The listing builds one solid part. Answer for the finished solid, in the listing's coordinates (mm). A direction names the side the tool comes from. Round coordinates to 2 decimals unless told otherwise and drop trailing zeros. Order: outer loops, then holes, each group sorted by start corner. A loop starts at its lowest first (then second) coordinate and runs counter-clockwise, first axis right, second up. Notation, with made-up numbers: (40, 31) -> (91, 31) arc R15 cw to (91, 46) -> close; hole circle Ø11 at (40, -1.75). An arc over 180 degrees is marked (long way). Answer in a Markdown table with one row per item. Add a question column.
```python
from build123d import *

# Parameters (mm, degrees)
SKETCH2_R           = 1.25
BOSS_EXTRUDE1_DEPTH = 69
SKETCH3_W           = 62
SKETCH3_H           = 4.5
CUT_EXTRUDE1_DEPTH  = 113.504444357
SKETCH4_W           = 54.406446317
SKETCH4_H           = 2.417375431
BOSS_EXTRUDE2_DEPTH = 83
FILLET1_R           = 1.5
FILLET2_R           = 2.5
FILLET3_R           = 1.5
CUT_EXTRUDE3_DEPTH  = 113.504444497
CUT_EXTRUDE5_REACH  = 114.504
SKETCH7_W           = 35
SKETCH7_H           = 3.5


with BuildPart() as part:
    # Sketch2 → Boss-Extrude1 (new body)
    with BuildSketch(Plane.XY):
        Polygon((0, 0), (0, 8), (88.5, 8), (88.5, 2.5), (85, 0), align=None)
        with Locations((6.000001876, 4)):
            Circle(SKETCH2_R, mode=Mode.SUBTRACT)
        with Locations((79.120881892, 4)):
            Circle(SKETCH2_R, mode=Mode.SUBTRACT)
    extrude(amount=BOSS_EXTRUDE1_DEPTH)

    # Sketch3 → Cut-Extrude1 (cut, through all)
    with BuildSketch(Plane.ZY):
        with Locations((34.5, 5.75)):
            Rectangle(SKETCH3_W, SKETCH3_H)
    extrude(amount=-CUT_EXTRUDE1_DEPTH, mode=Mode.SUBTRACT)

    # Sketch4 → Boss-Extrude2 (add)
    with BuildSketch(Plane.ZY):
        with Locations((34.04742318, 2.291312285)):
            Rectangle(SKETCH4_W, SKETCH4_H)
    extrude(amount=-BOSS_EXTRUDE2_DEPTH)

    # Fillet1
    fillet1_edges = [part.edges().sort_by_distance(p)[0] for p in [
        (42.5, 0, 69),
        (42.5, 0, 0),
    ]]
    fillet(fillet1_edges, radius=FILLET1_R)

    # Fillet2
    # the kernel refuses this fillet: 2.5 mm, written as the material it adds along each edge
    with BuildSketch(Plane(origin=(0, 3.5, 65.5), x_dir=(0, 0, -1), z_dir=(1, 0, 0))) as fillet2_piece_1_section:
        with BuildLine():
            CenterArc((FILLET2_R, FILLET2_R), FILLET2_R, 180, 90)
            Line((0, FILLET2_R), (0, 0))
            Line((0, 0), (FILLET2_R, 0))
        make_face()
    fillet2_piece_1 = extrude(amount=11.104357952, mode=Mode.PRIVATE)
    fillet2_piece_1 = fillet2_piece_1 - Plane(origin=(6.000001876, 4, 63.653309705), x_dir=(1, 0, 0), z_dir=(0, 0, -1)) * Cylinder(1.25, 33, mode=Mode.PRIVATE)
    add(fillet2_piece_1)
    with BuildSketch(Plane(origin=(0.8956458, 3.5, 65.5), x_dir=(0, 0, -1), z_dir=(1, 0, 0))) as fillet2_piece_2_section:
        with BuildLine():
            CenterArc((FILLET2_R, FILLET2_R), FILLET2_R, 180, 90)
            Line((0, FILLET2_R), (0, 0))
            Line((0, 0), (FILLET2_R, 0))
        make_face()
    fillet2_piece_2 = extrude(amount=83.329592169, mode=Mode.PRIVATE)
    fillet2_piece_2 = fillet2_piece_2 - Plane(origin=(6.000001876, 4, 64.936218349), x_dir=(1, 0, 0), z_dir=(0, 0, -1)) * Cylinder(1.25, 177, mode=Mode.PRIVATE)
    fillet2_piece_2 = fillet2_piece_2 - Plane(origin=(79.120881892, 4, 64.936218349), x_dir=(1, 0, 0), z_dir=(0, 0, -1)) * Cylinder(1.25, 177, mode=Mode.PRIVATE)
    add(fillet2_piece_2)
    with BuildSketch(Plane(origin=(0, 3.5, 3.5), x_dir=(0, 1, 0), z_dir=(1, 0, 0))) as fillet2_piece_3_section:
        with BuildLine():
            CenterArc((FILLET2_R, FILLET2_R), FILLET2_R, 180, 90)
            Line((0, FILLET2_R), (0, 0))
            Line((0, 0), (FILLET2_R, 0))
        make_face()
    fillet2_piece_3 = extrude(amount=11.104357952, mode=Mode.PRIVATE)
    fillet2_piece_3 = fillet2_piece_3 - Plane(origin=(6.000001876, 4, 3.561814983), x_dir=(1, 0, 0), z_dir=(0, 0, -1)) * Cylinder(1.25, 33, mode=Mode.PRIVATE)
    add(fillet2_piece_3)
    with BuildSketch(Plane(origin=(74.016525816, 3.5, 3.5), x_dir=(0, 1, 0), z_dir=(1, 0, 0))) as fillet2_piece_4_section:
        with BuildLine():
            CenterArc((FILLET2_R, FILLET2_R), FILLET2_R, 180, 90)
            Line((0, FILLET2_R), (0, 0))
            Line((0, 0), (FILLET2_R, 0))
        make_face()
    fillet2_piece_4 = extrude(amount=14.483474184, mode=Mode.PRIVATE)
    fillet2_piece_4 = fillet2_piece_4 - Plane(origin=(79.120881892, 4, 4.058892955), x_dir=(1, 0, 0), z_dir=(0, 0, -1)) * Cylinder(1.25, 39, mode=Mode.PRIVATE)
    add(fillet2_piece_4)
    with BuildSketch(Plane(origin=(0.8956458, 3.5, 3.5), x_dir=(0, 1, 0), z_dir=(1, 0, 0))) as fillet2_piece_5_section:
        with BuildLine():
            CenterArc((FILLET2_R, FILLET2_R), FILLET2_R, 180, 90)
            Line((0, FILLET2_R), (0, 0))
            Line((0, 0), (FILLET2_R, 0))
        make_face()
    fillet2_piece_5 = extrude(amount=83.329592169, mode=Mode.PRIVATE)
    fillet2_piece_5 = fillet2_piece_5 - Plane(origin=(79.120881892, 4, 4.063781674), x_dir=(1, 0, 0), z_dir=(0, 0, -1)) * Cylinder(1.25, 177, mode=Mode.PRIVATE)
    fillet2_piece_5 = fillet2_piece_5 - Plane(origin=(6.000001876, 4, 4.063781674), x_dir=(1, 0, 0), z_dir=(0, 0, -1)) * Cylinder(1.25, 177, mode=Mode.PRIVATE)
    add(fillet2_piece_5)
    with BuildSketch(Plane(origin=(74.016525816, 3.5, 65.5), x_dir=(0, 0, -1), z_dir=(1, 0, 0))) as fillet2_piece_6_section:
        with BuildLine():
            CenterArc((FILLET2_R, FILLET2_R), FILLET2_R, 180, 90)
            Line((0, FILLET2_R), (0, 0))
            Line((0, 0), (FILLET2_R, 0))
        make_face()
    fillet2_piece_6 = extrude(amount=14.483474184, mode=Mode.PRIVATE)
    fillet2_piece_6 = fillet2_piece_6 - Plane(origin=(79.120881892, 4, 64.941107203), x_dir=(1, 0, 0), z_dir=(0, 0, -1)) * Cylinder(1.25, 39, mode=Mode.PRIVATE)
    add(fillet2_piece_6)

    # Fillet3
    fillet3_edges = [part.edges().sort_by_distance(p)[0] for p in [
        (44.25, 8, 3.5),
        (44.25, 8, 65.5),
    ]]
    fillet(fillet3_edges, radius=FILLET3_R)

    # Sketch6 → Cut-Extrude3 (cut, through all)
    with BuildSketch(Plane.XZ):
        Polygon((-1.398299913, 8.05064563), (2.800616001, 8.05064563), (3.736645897, 7.027940595), (3.736645897, 1.098360778), (3.736645897, 0), (-1.236121559, -1.139461127), align=None)
    extrude(amount=-CUT_EXTRUDE3_DEPTH, mode=Mode.SUBTRACT)

    # Sketch7 → Cut-Extrude5 (cut, up to next)
    with BuildSketch(Plane.XZ, mode=Mode.PRIVATE) as cut_extrude5_sk1:
        with Locations((50, 56.69585569)):
            Rectangle(SKETCH7_W, SKETCH7_H)
    cut_extrude5_tool1 = extrude(cut_extrude5_sk1.sketch, amount=-CUT_EXTRUDE5_REACH, mode=Mode.PRIVATE) & part.part
    # Sketch7 → Cut-Extrude5 (cut, up to next)
    with BuildSketch(Plane.XZ, mode=Mode.PRIVATE) as cut_extrude5_sk2:
        with Locations((50, 11.19585569)):
            Rectangle(SKETCH7_W, SKETCH7_H)
    cut_extrude5_tool2 = extrude(cut_extrude5_sk2.sketch, amount=-CUT_EXTRUDE5_REACH, mode=Mode.PRIVATE) & part.part
    add(cut_extrude5_tool1.solids().sort_by_distance((50, 0, 56.695856))[0], mode=Mode.SUBTRACT)
    add(cut_extrude5_tool2.solids().sort_by_distance((50, 0, 11.195856))[0], mode=Mode.SUBTRACT)


solid = part.part
```
1. The part is cut by section B-B (z = 17.5). Give the vertices of the cut face in (x, y), then the cut area to 3 significant figures.
2. For faces 1 (the flat face through (44, 3.5, 34)), 2 (the cylindrical face through (79.617, 2.853, 65.932)), 3 (the cylindrical face through (79.617, 2.853, 2.614)), 4 (the flat face through (32.5, 2, 11)), 5 (the flat face through (1, 2, 8.051)), determine the directions among +Z, -Z, +X, -X, +Y, -Y from which every point of the face is accessible in a straight line to the end or side of a thin tool.
3. Straight lines are drawn through the part: line 1 along X through (y, z) = (4, 65); line 2 along X through (y, z) = (4, 3); line 3 along Z through (x, y) = (30, 6). For each, find the intervals that lie inside material, in ascending order.
4. The part is cut by section C-C (z = 64). Give the vertices of the cut face in (x, y).
5. The part is cut by section A-A (x = 26). Give the vertices of the cut face in (y, z), then the cut area to 3 significant figures.
6. The mould has two halves that part along Y. Classify faces 6 (the flat face through (50, 2, 9.446)), 7 (the cylindrical face through (6.496, 2.853, 2.614)), 8 (the flat face through (43, 0, 34)): released by +Y, released by -Y, zero draft, split by the parting line, or undercut.
7. This flat-tipped pin is pushed along its axis until it touches: pin 1 (2 mm diameter, centred on x = 79.12, y = 4, fed in from +Z). Where does it stop, or does it pass through?
Report:
| question | item | result |
|---|---|---|
| 1 | outline | (0, 0) -> (85, 0) -> (88.5, 2.5) -> (88.5, 3.5) -> (0, 3.5) -> close |
| 1 | area | 305 mm^2 |
| 2 | face 1 | +X, -X, +Y |
| 2 | face 2 | +Z |
| 2 | face 3 | -Z |
| 2 | face 4 | +Y, -Y |
| 2 | face 5 | -Z, -X, +Y, -Y |
| 3 | line 1 | x = 0 to 4.75, 7.25 to 77.87, 80.37 to 88.5 |
| 3 | line 2 | x = 3.74 to 4.75, 7.25 to 77.87, 80.37 to 88.5 |
| 3 | line 3 | z = 0 to 3.5, 65.5 to 69 |
| 4 | outline | (0, 0) -> (85, 0) -> (88.5, 2.5) -> (88.5, 3.71) -> (80.34, 3.71) arc R1.25 cw to (77.91, 3.71) -> (7.22, 3.71) arc R1.25 cw to (4.78, 3.71) -> (0, 3.71) -> close |
| 5 | outline | (0, 1.5) arc R1.5 ccw to (1.5, 0) -> (8, 0) -> (8, 2) arc R1.5 ccw to (6.5, 3.5) -> (6, 3.5) arc R2.5 cw to (3.5, 6) -> (3.5, 63) arc R2.5 cw to (6, 65.5) -> (6.5, 65.5) arc R1.5 ccw to (8, 67) -> (8, 69) -> (1.5, 69) arc R1.5 ccw to (0, 67.5) -> close |
| 5 | area | 274 mm^2 |
| 6 | face 6 | zero draft |
| 6 | face 7 | undercut |
| 6 | face 8 | released by -Y |
| 7 | pin 1 | stops at z = 61.25 |
